from build123d import *

# Parameters (mm, degrees)
F0_W     = 2
F0_H     = 26.25
F1_DEPTH = 4.2
F2_DEPTH = 1.2


with BuildPart() as f1:
    # F0 (on Top) → F1 (new body)
    with BuildSketch(Plane.XY):
        Polygon((21.05, -15.125), (21.05, 15.125), (5.55, 15.125), (5.55, 13.125), (19.05, 13.125), (19.05, -13.125), (-0.95, -13.125), (-0.95, -15.125), align=None)
        with Locations((-20.05, 0)):
            Rectangle(F0_W, F0_H)
    extrude(amount=F1_DEPTH)

    # F0 (on Top) → F2 (join)
    with BuildSketch(Plane.XY):
        Polygon((19.05, 13.125), (5.55, 13.125), (0.55, 13.125), (-19.05, 13.125), (-19.05, -13.125), (-0.95, -13.125), (19.05, -13.125), align=None)
    extrude(amount=F2_DEPTH)


solid = f1.part
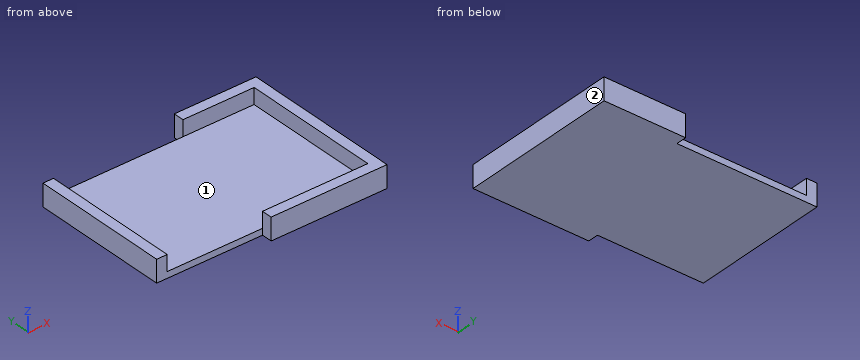
Source: CAD feature listing. Evaluate the final solid. Frame: model axes, mm. Face numbers are marked on the shaded views. A direction names the side the tool comes from. Give positions to 0.01 mm unless a question says otherwise; leave off trailing zeros. Write each loop counter-clockwise with the first axis right and the second up, starting at its lowest first coordinate (ties: lowest second). Pieces come first, ordered by that corner, then holes. Notation, with made-up numbers: (49, 81) -> (67, 81) arc R16 cw to (67, 89) -> close; hole circle Ø5 at (-7.5, -30). An arc over 180 degrees is marked (long way). Return JSON: item names as keys, results as strings. Group by question number.
1. Access query for the marked faces 1 and 2. Directions: +Z, -Z, +X, -X, +Y, -Y. A direction counts if a zero-diameter tool reaches every point of the face in a straight line with its end or side. Return the directions, or none.
2. Pin query (flat end, axial travel): pin 1 Ø1.6 at (y, z) = (14, 3) entering from -X; pin 2 Ø8 at (x, y) = (-8, 3.5) entering from +Z; pin 3 Ø1.6 at (y, z) = (-14, 2.5) entering from -X. Return the tip coordinate at first contact, or that it passes through.
3. Section A-A, the plane z = 2.05. Output: boundary loops of the cut face in (x, y) (3 decimals), then the cut area to 3 significant figures.
4. Section B-B, the plane y = 2.5. Output: boundary loops of the cut face in (x, z).
5. Section D-D, the plane x = 5. Output: boundary loops of the cut face in (y, z) (3 decimals).
6. Section C-C, the plane x = 16.5. Output: boundary loops of the cut face in (y, z) (3 decimals).
7. Material intervals for line 1 (X direction, y = 1, z = 3.2); line 2 (Y direction, x = 17, z = 3) (3 decimals); line 3 (Z direction, x = -11.5, y = -5), sorted ascending. Write a range as from..to.
Determined:
{
 "1": {"face 1": "+Z", "face 2": "+Z, -Z, +X, +Y, -Y"},
 "2": {"pin 1": "stops at x = 5.55", "pin 2": "stops at z = 1.2", "pin 3": "stops at x = -0.95"},
 "3": {"outline": "(-21.05, -13.125) -> (-19.05, -13.125) -> (-19.05, 13.125) -> (-21.05, 13.125) -> close; (-0.95, -15.125) -> (21.05, -15.125) -> (21.05, 15.125) -> (5.55, 15.125) -> (5.55, 13.125) -> (19.05, 13.125) -> (19.05, -13.125) -> (-0.95, -13.125) -> close", "area": "180 mm2"},
 "4": {"outline": "(-21.05, 0) -> (21.05, 0) -> (21.05, 4.2) -> (19.05, 4.2) -> (19.05, 1.2) -> (-19.05, 1.2) -> (-19.05, 4.2) -> (-21.05, 4.2) -> close"},
 "5": {"outline": "(-15.125, 0) -> (13.125, 0) -> (13.125, 1.2) -> (-13.125, 1.2) -> (-13.125, 4.2) -> (-15.125, 4.2) -> close"},
 "6": {"outline": "(-15.125, 0) -> (15.125, 0) -> (15.125, 4.2) -> (13.125, 4.2) -> (13.125, 1.2) -> (-13.125, 1.2) -> (-13.125, 4.2) -> (-15.125, 4.2) -> close"},
 "7": {"line 1": "x = -21.05..-19.05, 19.05..21.05", "line 2": "y = -15.125..-13.125, 13.125..15.125", "line 3": "z = 0..1.2"}
}
